```python
from build123d import *

# Parameters (mm, degrees)
F0_W     = 69.85
F0_H     = 254
F1_DEPTH = 25.4
F2_W     = 55.55453
F2_H     = 7.407263
F2_H_2   = 8.641817
F2_H_3   = 9.25909
F2_H_4   = 8.024544
F2_W_2   = 56.171801
F2_H_5   = 9.259089
F2_W_3   = 57.406345
F2_H_6   = 8.641819
F2_H_7   = 8.024541
F2_H_8   = 9.961726
F2_W_4   = 56.789074
F2_H_9   = 9.25908
F2_H_10  = 8.02454
F2_H_11  = 12.962729
F3_DEPTH = 25.4
F4_R     = 3.5
F5_DEPTH = 30


with BuildPart() as f1:
    # F0 (on Front) → F1 (new body)
    with BuildSketch(Plane.XZ):
        with Locations((-0.601145, 60.209312)):
            Rectangle(F0_W, F0_H)
    extrude(amount=F1_DEPTH)

    # F2 (on face) → F3 (cut, through all)
    with BuildSketch(Plane(origin=(0, 0, 0), x_dir=(-1, 0, 0), z_dir=(0, 1, 0))):
        with Locations((0.600389, 144.356407)):
            Rectangle(F2_W, F2_H)
        with Locations((0.600389, 125.220966)):
            Rectangle(F2_W, F2_H_2)
        with Locations((0.600389, 106.394149)):
            Rectangle(F2_W, F2_H_3)
        with Locations((0.600389, 86.641431)):
            Rectangle(F2_W, F2_H_4)
        with Locations((0.600389, 68.431888)):
            Rectangle(F2_W, F2_H_2)
        with Locations((0.291754, 50.222348)):
            Rectangle(F2_W_2, F2_H_5)
        with Locations((-0.325518, 32.630081)):
            Rectangle(F2_W_3, F2_H_6)
        with Locations((0.291754, 15.655086)):
            Rectangle(F2_W_2, F2_H_7)
        with Locations((0.291754, -4.980863)):
            Rectangle(F2_W_2, F2_H_8)
        with Locations((-0.016883, -22.615812)):
            Rectangle(F2_W_4, F2_H_9)
        with Locations((-0.016883, -40.516714)):
            Rectangle(F2_W_4, F2_H_10)
        with Locations((-0.016883, -54.713981)):
            Rectangle(F2_W_4, F2_H_10)
        with Locations((0.291754, 167.504131)):
            Rectangle(F2_W_2, F2_H_11)
    extrude(amount=-F3_DEPTH, mode=Mode.SUBTRACT)

    # F4 (on face) → F5 (join)
    with BuildSketch(Plane.XZ.offset(25.4)):
        with Locations((-28.126128, 180.871427)):
            Circle(F4_R)
        with Locations((26.781848, 180.871427)):
            Circle(F4_R)
    extrude(amount=F5_DEPTH)


solid = f1.part
```
Can you work these out from the model? Positions are in its coordinate system, mm. A direction names the side the tool comes from. Give positions to 0.01 mm unless a question says otherwise; leave off trailing zeros. Loops run counter-clockwise (first coordinate to the right, second up) from the corner with the lowest first, then second, coordinate; pieces in that order, holes last. Notation, with made-up numbers: M 71.5,73 L 88.5,73 A16 cw 88.5,101 Z; hole C 9,33 d11. An arc over 180 degrees is marked long. One line per question, with ' | ' between items. Start each with the question number.
Q1. If we section it at D-D (z = 155): Please give me the cut outline in (x, y), plus the area to 3 significant figures.
Q2. If I drill on line 1 (X direction, y = -8, z = -37); line 2 (X direction, y = -17, z = 32); line 3 (Y direction, x = -20, z = 57.5), over which ranges is the centre line in solid material (lowest first)? Write a range as from..to.
Q3. For pin 1 Ø12 at (x, y) = (-16.5, -41.5) entering from +Z; pin 2 Ø8 at (x, z) = (22, -32) entering from -Y, each with a flat end and sliding along its axis, tell me the tip position at first contact or that it passes through.
Q4. For faces 1 (the flat face through (-28.378, -13, 144)), 2 (the flat face through (-1, -13, 187.209)), which set-ups out of +Z, -Z, +X, -X, +Y, -Y let a thin tool reach every point of the face, with its end or its side?
Q5. If we section it at A-A (z = -41.5): Please give me the cut outline in (x, y).
Q6. If we mould it in two halves opening along X, with no side actions, what happens to faces 3 (the flat face through (27.177, -13, 87)), 4 (the flat face through (27.794, -13, 50)), 5 (the flat face through (-1, -13, -66.791))? For each: +X half, -X half, draft (parallel to the pull), parting line (faces both ways), or undercut.
Q7. If we section it at B-B (x = 13.5): State how many separate pieces and enclosed holes the cut face has, plus the area to 3 significant figures.
Computed:
1) outline: M -35.53,-25.4 L 34.32,-25.4 L 34.32,0 L -35.53,0 Z | area: 1,770 mm²
2) line 1: x = -35.53..-28.38, 28.41..34.32 | line 2: x = -35.53..-28.38, 29.03..34.32 | line 3: y = -25.4..0
3) pin 1: passes through | pin 2: stops at y = -25.4
4) face 1: +Y, -Y | face 2: +Z, +X, -X, +Y, -Y
5) outline: M -35.53,-25.4 L -28.38,-25.4 L -28.38,0 L -35.53,0 Z; M 28.41,-25.4 L 34.32,-25.4 L 34.32,0 L 28.41,0 Z
6) face 3: undercut | face 4: undercut | face 5: draft
7) separate pieces: 14 | enclosed holes: 0 | area: 3,500 mm²
